Read the model definition and answer for the solid it produces. Units are mm, in the model's axes. A direction names the side the tool comes from. Give positions to 0.01 mm unless a question says otherwise; leave off trailing zeros. Write each loop counter-clockwise with the first axis right and the second up, starting at its lowest first coordinate (ties: lowest second). Pieces come first, ordered by that corner, then holes. Notation, with made-up numbers: (24.5, 53) -> (52.5, 53) arc R22 ccw to (52.5, 59) -> close; hole circle Ø11 at (28.25, 57.5). An arc over 180 degrees is marked (long way). Answer as CSV lines item,"result". Start each with the question number.
1. The part is cut by section D-D, the plane z = 17. Determine the outline of the cut face in (x, y), and give its area (3 significant figures).
2. Find the intervals of material crossed by line 1 (Y direction, x = -6, z = 16.85); line 2 (X direction, y = -20.5, z = 16); line 3 (X direction, y = 14, z = 17.25), in increasing order.
3. The part is cut by section C-C, the plane y = 0.5. Determine the outline of the cut face in (x, z).
4. The part is cut by section B-B, the plane x = -76.5. Determine the outline of the cut face in (y, z).
5. For a pull along Y with two mould halves and no side action, classify faces 4 (the cylindrical face through (-29.458, -25.634, 14.489)), 5 (the cylindrical face through (-97.808, 15.242, 16.954)), 6 (the flat face through (-52, -17, 15.687)), 7 (the flat face through (-53, 8.367, 17)) as pulls with the +Y half, pulls with the -Y half, needs draft (parallel to the pull), parting line crosses it, or undercut.
6. The part is cut by section A-A, the plane x = -6. Determine the outline of the cut face in (y, z), and give its area (3 significant figures).
7. Given pin 1 (2 mm diameter, centred on x = -6, y = 14.87, fed in from +Z); pin 2 (23 mm diameter, centred on x = -44.5, y = -2, fed in from -Z); pin 3 (2.5 mm diameter, centred on y = -20.5, z = 13.5, fed in from -X); pin 4 (2.5 mm diameter, centred on x = -69, z = 13, fed in from +Y), each flat-ended and moving along its own axis, determine where each tip first touches the part or whether it passes through.
8. A tool of negligible diameter and unlimited length cuts with its end or side. For faces 1 (the flat face through (-1, -16.633, 13)), 2 (the flat face through (-2.5, -21, 13)), 3 (the flat face through (-16.099, -4, 17)), from which of +Z, -Z, +X, -X, +Y, -Y can it reach the whole face along a straight path? Write none if from no direction.
from build123d import *

# Parameters (mm, degrees)
F0_W     = 2.2
F0_H     = 5
F1_DEPTH = 105
F2_R     = 1.25
F3_DEPTH = 2.5
F4_W     = 71.900862
F4_H     = 25
F5_DEPTH = 7.5
F0_W_2   = 8
F6_DEPTH = 2.5


with BuildPart() as f1:
    # F0 (on Right) → F1 (new body)
    with BuildSketch(Plane.YZ):
        with Locations((-25.733312, 13.186514)):
            Rectangle(F0_W, F0_H)
        Polygon((-26.833312, 15.686514), (-24.633312, 15.686514), (-16.633312, 15.686514), (21.366688, 15.686514), (21.366688, 18.186514), (-26.833312, 18.186514), align=None)
    extrude(amount=-F1_DEPTH)

    # F2 (on face) → F3 (cut)
    with BuildSketch(Plane.XY.offset(18.186514)):
        with Locations((-99, 14.866688)):
            Circle(F2_R)
        with Locations((-6, 14.866688)):
            Circle(F2_R)
        with Locations((-6, -20.333312)):
            Circle(F2_R)
        with Locations((-99, -20.333312)):
            Circle(F2_R)
    extrude(amount=-F3_DEPTH, mode=Mode.SUBTRACT)

    # F4 (on face) → F5 (cut)
    with BuildSketch(Plane.XY.offset(18.186514)):
        with Locations((-52.049569, -4.133312)):
            Rectangle(F4_W, F4_H)
        with BuildLine():
            Line((-32.138181, -26.833312), (-26.861819, -26.833312))
            ThreePointArc((-26.861819, -26.833312), (-29.5, -25.633312), (-32.138181, -26.833312))
        make_face()
    extrude(amount=-F5_DEPTH, mode=Mode.SUBTRACT)

    # F0 (on Right) → F6 (join)
    with BuildSketch(Plane.YZ):
        with Locations((-20.633312, 13.186514)):
            Rectangle(F0_W_2, F0_H)
    extrude(amount=-F6_DEPTH)


solid = f1.part
Results found:
1,outline,"(-105, -26.83) -> (-32.14, -26.83) arc R3.5 cw to (-26.86, -26.83) -> (0, -26.83) -> (0, 21.37) -> (-105, 21.37) -> close; hole circle Ø2.5 at (-99, -20.33); hole circle Ø2.5 at (-99, 14.87); hole (-88, -16.63) -> (-16.1, -16.63) -> (-16.1, 8.37) -> (-88, 8.37) -> close; hole circle Ø2.5 at (-6, -20.33); hole circle Ø2.5 at (-6, 14.87)"
1,area,"3,240 mm²"
2,line 1,"y = -26.83 to -21.58, -19.08 to 13.62, 16.12 to 21.37"
2,line 2,"x = -105 to -100.24, -97.76 to -7.24, -4.76 to 0"
2,line 3,"x = -105 to -99.9, -98.1 to -6.9, -5.1 to 0"
3,outline,"(-105, 15.69) -> (-88, 15.69) -> (-88, 18.19) -> (-105, 18.19) -> close; (-16.1, 15.69) -> (0, 15.69) -> (0, 18.19) -> (-16.1, 18.19) -> close"
4,outline,"(-26.83, 10.69) -> (-24.63, 10.69) -> (-24.63, 15.69) -> (-16.63, 15.69) -> (-16.63, 18.19) -> (-26.83, 18.19) -> close; (8.37, 15.69) -> (21.37, 15.69) -> (21.37, 18.19) -> (8.37, 18.19) -> close"
5,face 4,"pulls with the -Y half"
5,face 5,"undercut"
5,face 6,"needs draft"
5,face 7,"undercut"
6,outline,"(-26.83, 10.69) -> (-24.63, 10.69) -> (-24.63, 15.69) -> (-21.58, 15.69) -> (-21.58, 18.19) -> (-26.83, 18.19) -> close; (-19.08, 15.69) -> (13.62, 15.69) -> (13.62, 18.19) -> (-19.08, 18.19) -> close; (16.12, 15.69) -> (21.37, 15.69) -> (21.37, 18.19) -> (16.12, 18.19) -> close"
6,area,"119 mm²"
7,pin 1,"passes through"
7,pin 2,"stops at z = 15.69"
7,pin 3,"stops at x = -2.5"
7,pin 4,"stops at y = -24.63"
8,face 1,"-Z, +X, -X, +Y"
8,face 2,"-Z, -X, +Y"
8,face 3,"+Z, -Z"
